from build123d import *

# Parameters (mm, degrees)
F0_W     = 130
F0_H     = 120
F2_DEPTH = 3
F1_W     = 3
F1_H     = 10
F3_DEPTH = 25
F4_W     = 10
F4_H     = 3
F5_DEPTH = 25
F6_W     = 3
F6_H     = 10
F7_DEPTH = 25


with BuildPart() as f2:
    # F0 (on Top) → F2 (new body)
    with BuildSketch(Plane.XY):
        Rectangle(F0_W, F0_H)
    extrude(amount=F2_DEPTH)

    # F1 (on face) → F3 (cut)
    with BuildSketch(Plane.XY):
        with Locations((63.5, -55)):
            Rectangle(F1_W, F1_H)
        with Locations((63.5, -35)):
            Rectangle(F1_W, F1_H)
        with Locations((63.5, -15)):
            Rectangle(F1_W, F1_H)
        with Locations((63.5, 5)):
            Rectangle(F1_W, F1_H)
        with Locations((63.5, 25)):
            Rectangle(F1_W, F1_H)
        with Locations((63.5, 45)):
            Rectangle(F1_W, F1_H)
        with Locations((-63.5, -55)):
            Rectangle(F1_W, F1_H)
        with Locations((-63.5, 25)):
            Rectangle(F1_W, F1_H)
        with Locations((-63.5, 5)):
            Rectangle(F1_W, F1_H)
        with Locations((-63.5, -15)):
            Rectangle(F1_W, F1_H)
        with Locations((-63.5, 45)):
            Rectangle(F1_W, F1_H)
        with Locations((-63.5, -35)):
            Rectangle(F1_W, F1_H)
    extrude(amount=F3_DEPTH, mode=Mode.SUBTRACT)

    # F4 (on face) → F5 (cut)
    with BuildSketch(Plane.XY.offset(3)):
        with Locations((-50, -58.5)):
            Rectangle(F4_W, F4_H)
        with Locations((-30, -58.5)):
            Rectangle(F4_W, F4_H)
        with Locations((-10, -58.5)):
            Rectangle(F4_W, F4_H)
        with Locations((10, -58.5)):
            Rectangle(F4_W, F4_H)
        with Locations((30, -58.5)):
            Rectangle(F4_W, F4_H)
        with Locations((50, -58.5)):
            Rectangle(F4_W, F4_H)
    extrude(amount=-F5_DEPTH, mode=Mode.SUBTRACT)

    # F6 (on face) → F7 (cut)
    with BuildSketch(Plane.XY.offset(3)):
        with Locations((63.5, 55)):
            Rectangle(F6_W, F6_H)
        with Locations((-63.5, 55)):
            Rectangle(F6_W, F6_H)
    extrude(amount=-F7_DEPTH, mode=Mode.SUBTRACT)


solid = f2.part
For this review, take the finished solid that the model builds, in its own axes (mm). A direction names the side the tool comes from. Round coordinates to 2 decimals unless told otherwise and drop trailing zeros. Order: outer loops, then holes, each group sorted by start corner. A loop starts at its lowest first (then second) coordinate and runs counter-clockwise, first axis right, second up. Notation, with made-up numbers: M -3.5,-23.5 L 55.5,-23.5 A21 ccw 55.5,4.5 Z; hole C 51.5,-36.5 d5. An arc over 180 degrees is marked long. Write each question's results on one line, items separated by ' | '. Start each with the question number.
1. Tool access review of faces 4 (the face through (63, -10, 1)), 5 (the face through (-62, -55, 1)), 6 (the face through (15, -59, 2)), 7 (the face through (62, 50, 2)), 8 (the face through (-64, -20, 1)): name each direction out of +Z, -Z, +X, -X, +Y, -Y from which nothing blocks a thin tool from reaching the whole face with its end or side.
2. To check wall thickness, follow L1, parallel to Y at x = -9, z = 0.5; L2, parallel to X at y = 3, z = 2.85. State the ranges of each line that lie inside material, in increasing order. Write a range as [from, to].
3. Add section B-B (y = -16.5). State the section outline as (x, z) points.
4. Clearance check with flat-ended pins moving along their axes: pin 1 Ø2 at (x, y) = (4.5, -38) entering from -Z; pin 2 Ø1.5 at (y, z) = (-58.5, 2) entering from -X; pin 3 Ø1.5 at (y, z) = (-15, 1.5) entering from +X; pin 4 Ø1 at (x, z) = (-50.5, 2) entering from -Y. State where each tip first meets the part, or that it passes through.
5. Add section A-A (x = 49.5). State the section outline as (y, z) points, then the cut area to 3 significant figures.
6. Draft analysis for pull direction Y (two halves, no side actions). For faces 1 (the face through (-62, -15, 1)), 2 (the face through (63, -50, 1)), 3 (the face through (-35, -59, 2)), state which applies: pulls with the +Y half, pulls with the -Y half, needs draft (parallel to the pull), parting line crosses it, or undercut.
Output values:
1) face 4: +Z, -Z, +X | face 5: +Z, -Z, -X, -Y | face 6: +Z, -Z, -Y | face 7: +Z, -Z, +X, +Y | face 8: +Z, -Z, -X
2) L1: [-57, 60] | L2: [-62, 62]
3) outline: M -62,0 L 62,0 L 62,3 L -62,3 Z
4) pin 1: z = 0 | pin 2: x = -62 | pin 3: x = 62 | pin 4: y = -57
5) outline: M -57,0 L 60,0 L 60,3 L -57,3 Z | area: 351 mm^2
6) face 1: undercut | face 2: pulls with the -Y half | face 3: needs draft
